Part model, mm, in its own coordinate system. Round coordinates to 2 decimals unless told otherwise and drop trailing zeros. Order: outer loops, then holes, each group sorted by start corner. A loop starts at its lowest first (then second) coordinate and runs counter-clockwise, first axis right, second up. Notation, with made-up numbers: (83.5, 38) -> (136.5, 38) arc R12 cw to (136.5, 56) -> close; hole circle Ø2 at (28, 4). An arc over 180 degrees is marked (long way). Use CSV: the item, a comma, the result in double quotes.
```python
from build123d import *

# Parameters (mm, degrees)
F0_R     = 9.525
F1_DEPTH = 25.4
F2_SIZE  = 0.508
F3_T     = -0.508


with BuildPart() as f1:
    # F0 (on Top) → F1 (new body)
    with BuildSketch(Plane.XY):
        Circle(F0_R)
    extrude(amount=F1_DEPTH)

    # F2
    f2_edges = [f1.edges().sort_by_distance(p)[0] for p in [
        (-9.525, 0, 25.4),
    ]]
    chamfer(f2_edges, length=F2_SIZE)

    # F3
    f3_openings = [f1.faces().sort_by_distance(p)[0] for p in [
        (0, 0, 0),
    ]]
    offset(amount=F3_T, openings=f3_openings)


solid = f1.part
```
(1) Cut at A-A, the plane x = 0. Give the cut face in (y, z) (3 decimals).
Reply:
outline,"(-9.525, 0) -> (-9.017, 0) -> (-9.017, 24.682) -> (-8.807, 24.892) -> (8.807, 24.892) -> (9.017, 24.682) -> (9.017, 0) -> (9.525, 0) -> (9.525, 24.892) -> (9.017, 25.4) -> (-9.017, 25.4) -> (-9.525, 24.892) -> close"
(2) Cut at C-C, the plane z = 3.75. Give the cut face in (x, y) (3 decimals).
Reply:
outline,"circle Ø19.05 at (0, 0); hole circle Ø18.034 at (0, 0)"
(3) Drop flat-ended pins along their axis: P1, Ø6, axis at y = -5.5, z = 20.5, coming from the +X side; P2, Ø4, axis at x = -4, z = 20.5, coming from the -Y side; P3, Ø1.5, axis at x = 5.5, z = 3.5, coming from the -Y side. Give the stop position or say it passes through.
Reply:
P1,"x = 9.19"
P2,"y = -9.31"
P3,"y = -8.26"
(4) Probe probe 1 along Y at (x, z) = (-0.25, 24); probe 2 along Z at (x, y) = (8, 3.5); probe 3 along X at (y, z) = (-3.5, 14.75). List the from-to ranges inside material, lowest first. Write a range as [from, to].
Reply:
probe 1,"[-9.52, -9.01], [9.01, 9.52]"
probe 2,"[24.89, 25.4]"
probe 3,"[-8.86, -8.31], [8.31, 8.86]"
(5) Pull direction X, two halves, no side cores. Call faces 1 (the face through (-7.559, -5.796, 12.272)), 2 (the face through (-1.955, -8.803, 12.168)), 3 (the face through (0, 0, 24.892)), 4 (the face through (0, 0, 25.4)): released by +X, released by -X, zero draft, split by the parting line, or undercut.
Reply:
face 1,"split by the parting line"
face 2,"undercut"
face 3,"undercut"
face 4,"zero draft"
